from build123d import *

# Parameters (mm, degrees)
SKETCH1_W           = 58.42
SKETCH1_H           = 34.29
SKETCH1_W_2         = 22.86
SKETCH1_H_2         = 24.13
SKETCH1_H_3         = 25.4
BOSS_EXTRUDE1_DEPTH = 63.5
SKETCH2_W           = 58.42
SKETCH2_H           = 59.69
BOSS_EXTRUDE2_DEPTH = 2.54
SKETCH3_R           = 2.54
CUT_EXTRUDE1_DEPTH  = 84.81278378
SKETCH6_W           = 54.61
SKETCH6_H           = 20.828
CUT_EXTRUDE3_DEPTH  = 9.979406
SKETCH7_R           = 2.2352
CUT_EXTRUDE4_DEPTH  = 12.7
SKETCH9_W           = 41.91
SKETCH9_H           = 20.574
CUT_EXTRUDE5_DEPTH  = 27.94
SKETCH10_R          = 6.096
CUT_EXTRUDE6_DEPTH  = 94.208829249
CUT_EXTRUDE7_DEPTH  = 92.374500249
CHAMFER1_SIZE       = 1.778


with BuildPart() as part:
    # Sketch1 → Boss-Extrude1 (new body)
    # profile 1 of 2: a face of its own
    with BuildSketch(Plane(origin=(0, 0, 0), x_dir=(1, 0, 0), z_dir=(0, 1, 0))):
        Rectangle(SKETCH1_W, SKETCH1_H)
        with Locations((-12.7, 0)):
            Rectangle(SKETCH1_W_2, SKETCH1_H_2, mode=Mode.SUBTRACT)
        with Locations((12.7, 0)):
            Rectangle(SKETCH1_W_2, SKETCH1_H_2, mode=Mode.SUBTRACT)
    # profile 2 of 2: a face of its own
    with BuildSketch(Plane(origin=(0, 0, 0), x_dir=(1, 0, 0), z_dir=(0, 1, 0))):
        with Locations((0, -29.845)):
            Rectangle(SKETCH1_W, SKETCH1_H_3)
    extrude(amount=BOSS_EXTRUDE1_DEPTH)

    # Sketch2 → Boss-Extrude2 (add)
    with BuildSketch(Plane(origin=(0, 63.5, 0), x_dir=(1, 0, 0), z_dir=(0, 1, 0))):
        with Locations((0, -12.7)):
            Rectangle(SKETCH2_W, SKETCH2_H)
    extrude(amount=BOSS_EXTRUDE2_DEPTH)

    # Sketch3 → Cut-Extrude1 (cut, through all)
    with BuildSketch(Plane(origin=(0, 66.04, 0), x_dir=(1, 0, 0), z_dir=(0, 1, 0))):
        with Locations(Location((-19.05, 0, 0), (0, 0, 270))):
            Circle(SKETCH3_R)
        with Locations(Location((19.05, 0, 0), (0, 0, 270))):
            Circle(SKETCH3_R)
    extrude(amount=-CUT_EXTRUDE1_DEPTH, mode=Mode.SUBTRACT)

    # Sketch6 → Cut-Extrude3 (cut)
    with BuildSketch(Plane.XZ):
        with Locations((0, 28.557227446)):
            Rectangle(SKETCH6_W, SKETCH6_H)
    extrude(amount=-CUT_EXTRUDE3_DEPTH, mode=Mode.SUBTRACT)

    # Sketch7 → Cut-Extrude4 (cut)
    with BuildSketch(Plane.XZ.offset(-9.979406)):
        with Locations(Location((24.09, 36.930859788, 0), (0, 0, 270))):
            Circle(SKETCH7_R)
        with Locations(Location((24.09, 23.757367658, 0), (0, 0, 270))):
            Circle(SKETCH7_R)
        with Locations(Location((-24.09, 23.757367658, 0), (0, 0, 270))):
            Circle(SKETCH7_R)
        with Locations(Location((-24.09, 36.930859788, 0), (0, 0, 270))):
            Circle(SKETCH7_R)
    extrude(amount=-CUT_EXTRUDE4_DEPTH, mode=Mode.SUBTRACT)

    # Sketch9 → Cut-Extrude5 (cut)
    with BuildSketch(Plane.XZ.offset(-9.979406)):
        with Locations((0, 28.557227446)):
            Rectangle(SKETCH9_W, SKETCH9_H)
    extrude(amount=-CUT_EXTRUDE5_DEPTH, mode=Mode.SUBTRACT)

    # Sketch10 → Cut-Extrude6 (cut, through all)
    with BuildSketch(Plane(origin=(-20.955, 0, 0), x_dir=(0, 0, -1), z_dir=(1, 0, 0))):
        with Locations((-28.557227446, 26.477976)):
            Circle(SKETCH10_R)
    extrude(amount=-CUT_EXTRUDE6_DEPTH, mode=Mode.SUBTRACT)

    # Sketch11 → Cut-Extrude7 (cut, through all)
    with BuildSketch(Plane(origin=(0, 0, 38.844227446), x_dir=(-1, 0, 0), z_dir=(0, 0, -1))):
        Polygon((-27.305, 0), (27.305, 0), (27.305, 9.979406), (25.002698669, 9.979406), (23.177301331, 9.979406), (20.955, 9.979406), (20.955, 37.919406), (-20.955, 37.919406), (-20.955, 9.979406), (-23.177301331, 9.979406), (-25.002698669, 9.979406), (-27.305, 9.979406), align=None)
    extrude(amount=-CUT_EXTRUDE7_DEPTH, mode=Mode.SUBTRACT)

    # Chamfer1
    # the kernel refuses this chamfer: 1.778 mm, written as the material it takes off along each edge
    with BuildSketch(Plane(origin=(-20.955, 26.477976, 28.557227446), x_dir=(0, 0, -1), z_dir=(0, -1, 0))) as chamfer1_piece_1:
        Polygon((6.096, -CHAMFER1_SIZE), (6.096 + CHAMFER1_SIZE, 0), (6.096, 0), align=None)
    revolve(axis=Axis((-20.955, 26.477976, 28.557227446), (1, 0, 0)), mode=Mode.SUBTRACT)


solid = part.part
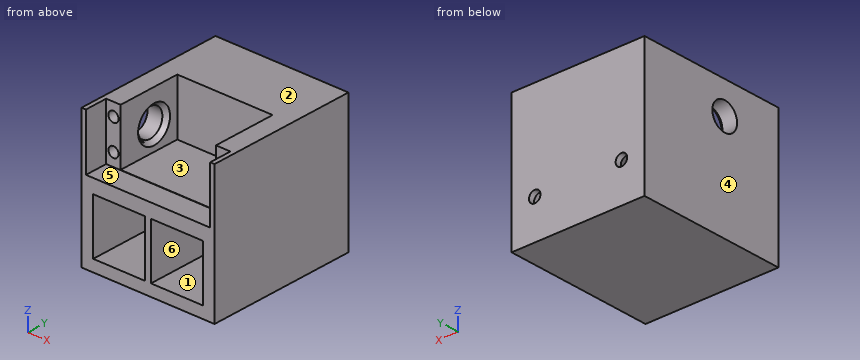
Read the model definition and answer for the solid it produces. Units are mm, in the model's axes. Face numbers are marked on the shaded views. A direction names the side the tool comes from. Coordinates: 2 decimals unless noted, no trailing zeros. Loops run counter-clockwise (first coordinate to the right, second up) from the corner with the lowest first, then second, coordinate; pieces in that order, holes last.
Q1. Consider probe 1 along X at (y, z) = (10, 3); probe 2 along Z at (x, y) = (19, 64) (1 decimal); probe 3 along Z at (x, y) = (-5.5, 44.5) (3 decimals). Determine where each line is inside the solid, lowest interval first.
Q2. Which of the six approach directions +Z, -Z, +X, -X, +Y, -Y give full straight-line access (tool end or side, diameter ignored) to the marked faces 1, 2 and 3?
Q3. The part is cut by section B-B on z = 0. Write down the section's boundary in (x, y).
Q4. The part is cut by section D-D on y = 47.5. Write down the section's boundary in (x, z) (3 decimals), and give its area (3 significant figures).
Q5. The mould has two halves that part along Z. Classify the marked faces 4, 5 and 6: +Z half, -Z half, draft (parallel to the pull), parting line (faces both ways), or undercut.
Q6. The part is cut by section C-C on x = 0. Write down the section's boundary in (y, z) (3 decimals), and give its area (3 significant figures).
Q7. Each of these flat-tipped pins is pushed along its axis until it touches: pin 1 Ø4 at (x, y) = (-7.5, 16.5) entering from +Z; pin 2 Ø6 at (x, z) = (-24.09, 23.76) entering from -Y; pin 3 Ø12 at (x, z) = (-17, 5) entering from -Y. Where does it stop, or does it pass through?
Q8. The part is cut by section A-A on x = 19.05. Write down the section's boundary in (y, z) (3 decimals).
Results below:
1. probe 1: x = -29.21 to -24.13, -1.27 to 1.27, 24.13 to 29.21
1. probe 2: z = -17.1 to -2.5, 2.5 to 42.5
1. probe 3: z = -17.145 to -12.065, 12.065 to 42.545
2. face 1: -Y
2. face 2: +Z, +X, -X, +Y, -Y
2. face 3: +Z, -Y
3. outline: (-29.21, 0) - (-24.13, 0) - (-24.13, 63.5) - (-21.59, 63.5) - (-21.59, 66.04) - (-29.21, 66.04) - close; (-16.51, 63.5) - (-1.27, 63.5) - (-1.27, 0) - (1.27, 0) - (1.27, 63.5) - (16.51, 63.5) - (16.51, 66.04) - (-16.51, 66.04) - close; (21.59, 63.5) - (24.13, 63.5) - (24.13, 0) - (29.21, 0) - (29.21, 66.04) - (21.59, 66.04) - close
4. outline: (-29.21, -17.145) - (29.21, -17.145) - (29.21, 42.545) - (-29.21, 42.545) - close; hole (-24.13, -12.065) - (-1.27, -12.065) - (-1.27, 12.065) - (-24.13, 12.065) - close; hole (1.27, -12.065) - (24.13, -12.065) - (24.13, 12.065) - (1.27, 12.065) - close
4. area: 2,380 mm2
5. face 4: draft
5. face 5: +Z half
5. face 6: undercut
6. outline: (0, -17.145) - (66.04, -17.145) - (66.04, 42.545) - (37.919, 42.545) - (37.919, 18.27) - (9.979, 18.27) - (9.979, 18.143) - (0, 18.143) - close
6. area: 3,020 mm2
7. pin 1: stops at z = 18.27
7. pin 2: stops at y = 9.98
7. pin 3: stops at y = 63.5
8. outline: (0, -17.145) - (66.04, -17.145) - (66.04, -2.54) - (63.5, -2.54) - (63.5, -12.065) - (0, -12.065) - close; (0, 12.065) - (63.5, 12.065) - (63.5, 2.54) - (66.04, 2.54) - (66.04, 42.545) - (37.919, 42.545) - (37.919, 18.27) - (9.979, 18.27) - (9.979, 18.143) - (0, 18.143) - close
